from build123d import *

# Parameters (mm, degrees)
SKETCH1_R           = 2.125
BOSS_EXTRUDE1_DEPTH = 3.175


with BuildPart() as part:
    # Sketch1 → Boss-Extrude1 (new body)
    with BuildSketch(Plane(origin=(0, 0, 0), x_dir=(1, 0, 0), z_dir=(0, 1, 0))):
        with BuildLine():
            Line((52.831908676, -29.265059171), (52.831908676, 26.025389594))
            ThreePointArc((52.831908676, 26.025389594), (53.463014101, 27.639628661), (55.021629488, 28.397771062))
            ThreePointArc((55.021629488, 28.397771062), (60.077505451, 34.100201776), (54.581908676, 39.380165211))
            Line((54.581908676, 39.380165211), (-66.918091324, 39.380165211))
            ThreePointArc((-66.918091324, 39.380165211), (-72.413688099, 34.100201776), (-67.357812136, 28.397771062))
            ThreePointArc((-67.357812136, 28.397771062), (-65.799196749, 27.639628661), (-65.168091324, 26.025389594))
            Line((-65.168091324, 26.025389594), (-65.168091324, -29.265059171))
            ThreePointArc((-65.168091324, -29.265059171), (-65.799196749, -30.879298239), (-67.357812136, -31.63744064))
            ThreePointArc((-67.357812136, -31.63744064), (-72.413688099, -37.339871353), (-66.918091324, -42.619834789))
            Line((-66.918091324, -42.619834789), (54.581908676, -42.619834789))
            ThreePointArc((54.581908676, -42.619834789), (60.077505451, -37.339871353), (55.021629488, -31.63744064))
            ThreePointArc((55.021629488, -31.63744064), (53.463014101, -30.879298239), (52.831908676, -29.265059171))
        make_face()
        with Locations(Location((-66.918091324, 33.880165211, 0), (0, 0, 270))):
            Circle(SKETCH1_R, mode=Mode.SUBTRACT)
        with Locations(Location((54.581908676, 33.880165211, 0), (0, 0, 270))):
            Circle(SKETCH1_R, mode=Mode.SUBTRACT)
        with Locations(Location((54.581908676, -37.119834789, 0), (0, 0, 270))):
            Circle(SKETCH1_R, mode=Mode.SUBTRACT)
        with Locations(Location((-66.918091324, -37.119834789, 0), (0, 0, 270))):
            Circle(SKETCH1_R, mode=Mode.SUBTRACT)
        with BuildLine():
            Line((40.163908241, -6.264833275), (42.163908241, -6.264833251))
            Line((42.163908241, -6.264833251), (42.16390822, -4.464833251))
            Line((42.16390822, -4.464833251), (40.16390822, -4.464833275))
            Line((40.16390822, -4.464833275), (40.163908156, 0.935166725))
            Line((40.163908156, 0.935166725), (42.163908156, 0.935166749))
            Line((42.163908156, 0.935166749), (42.163908134, 2.735166749))
            Line((42.163908134, 2.735166749), (40.163908134, 2.735166725))
            Line((40.163908134, 2.735166725), (40.163908003, 13.735166725))
            ThreePointArc((40.163908003, 13.735166725), (38.347969994, 18.119228747), (33.963907929, 19.935166651))
            Line((33.963907929, 19.935166651), (22.763907929, 19.935166518))
            ThreePointArc((22.763907929, 19.935166518), (18.379845907, 18.119228509), (16.563908003, 13.735166444))
            Line((16.563908003, 13.735166444), (16.563908373, -17.264833556))
            ThreePointArc((16.563908373, -17.264833556), (18.379846382, -21.648895578), (22.763908447, -23.464833482))
            Line((22.763908447, -23.464833482), (33.963908447, -23.464833349))
            ThreePointArc((33.963908447, -23.464833349), (38.347970468, -21.64889534), (40.163908373, -17.264833275))
            Line((40.163908373, -17.264833275), (40.163908241, -6.264833275))
        make_face(mode=Mode.SUBTRACT)
    extrude(amount=BOSS_EXTRUDE1_DEPTH)


solid = part.part
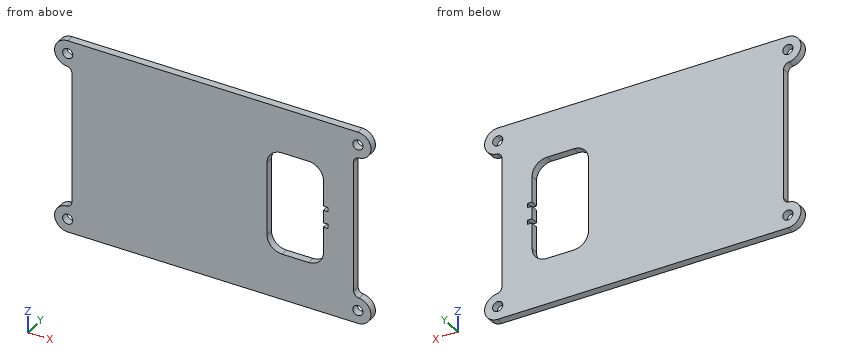
The listing builds one solid part. Answer for the finished solid, in the listing's coordinates (mm). Give positions to 0.01 mm unless a question says otherwise; leave off trailing zeros. Write each loop counter-clockwise with the first axis right and the second up, starting at its lowest first coordinate (ties: lowest second). Pieces come first, ordered by that corner, then holes. Notation, with made-up numbers: (-23.5, 26.25) - (-18.5, 26.25) arc R22 ccw to (-18.5, 47.25) - close; hole circle Ø1 at (44.25, -19.75). An arc over 180 degrees is marked (long way). Use a Markdown table: item, result.
1. Find the intervals of material crossed by probe 1 along Z at (x, y) = (41.5, 2); probe 2 along X at (y, z) = (0.9, -8); probe 3 along Z at (x, y) = (34, 0.5), in increasing order. Write a range as from..to.
Values follow:
| item | result |
|---|---|
| probe 1 | z = -39.38..-2.74, -0.94..4.46, 6.26..42.62 |
| probe 2 | x = -65.17..16.56, 40.16..52.83 |
| probe 3 | z = -39.38..-19.94, 23.46..42.62 |
2. Section B-B on y = 0.65 is taken. Count the separate pieces of the cut face and the enclosed holes in it, plus the area to 3 significant figures.
Values follow:
| item | result |
|---|---|
| separate pieces | 1 |
| enclosed holes | 5 |
| area | 8,890 mm² |
3. Section A-A on x = 27 is taken. Write down the section's boundary in (y, z) (3 decimals), plus the area to 3 significant figures.
Values follow:
| item | result |
|---|---|
| outline | (0, -39.38) - (3.175, -39.38) - (3.175, -19.935) - (0, -19.935) - close; (0, 23.465) - (3.175, 23.465) - (3.175, 42.62) - (0, 42.62) - close |
| area | 123 mm² |
4. Section C-C on z = -15.5 is taken. Write down the section's boundary in (x, y) (3 decimals).
Values follow:
| item | result |
|---|---|
| outline | (-65.168, 0) - (16.82, 0) - (16.82, 3.175) - (-65.168, 3.175) - close; (39.907, 0) - (52.832, 0) - (52.832, 3.175) - (39.907, 3.175) - close |
5. Each of these flat-tipped pins is pushed along its axis until it touches: P1, Ø1.4, axis at y = 2.5, z = -1.5, coming from the -X side; P2, Ø3.5, axis at x = -66.92, z = -33.88, coming from the -Y side. Where does it stop, or does it pass through?
Values follow:
| item | result |
|---|---|
| P1 | stops at x = -65.17 |
| P2 | passes through |
